CAD build for the part. Positions are in the model's coordinates, mm. A direction names the side the tool comes from. Round coordinates to 2 decimals unless told otherwise and drop trailing zeros. Loops run counter-clockwise (first coordinate to the right, second up) from the corner with the lowest first, then second, coordinate; pieces in that order, holes last.
```python
from build123d import *

# Parameters (mm, degrees)
F0_W     = 1.524
F0_H     = 6.35
F0_W_2   = 6.35
F0_H_2   = 1.524
F1_DEPTH = 1.524


with BuildPart() as f1:
    # F0 (on Front) → F1 (new body)
    with BuildSketch(Plane.XZ):
        Polygon((30.226, 19.05), (30.226, 25.4), (25.4, 25.4), (25.4, 21.0894770619), (25.4, -21.0894770619), (25.4, -25.4), (21.0894770619, -25.4), (-21.0894770619, -25.4), (-25.4, -25.4), (-25.4, -21.0894770619), (-25.4, 21.0894770619), (-25.4, 25.4), (-30.226, 25.4), (-30.226, 19.05), (-30.226, 12.7), (-30.226, -12.7), (-30.226, -19.05), (-30.226, -31.75), (-19.05, -31.75), (-12.7, -31.75), (12.7, -31.75), (19.05, -31.75), (30.226, -31.75), (30.226, -19.05), (30.226, -12.7), (30.226, 12.7), align=None)
        with Locations((-30.988, -15.875)):
            Rectangle(F0_W, F0_H)
        with Locations((-15.875, -32.512)):
            Rectangle(F0_W_2, F0_H_2)
        with Locations((15.875, -32.512)):
            Rectangle(F0_W_2, F0_H_2)
        Polygon((25.4, -25.4), (25.4, -21.0894770619), (4.3105229381, 0), (0, -4.3105229381), (21.0894770619, -25.4), align=None)
        Polygon((4.3105229381, 0), (0, 4.3105229381), (-4.3105229381, 0), (0, -4.3105229381), align=None)
        Polygon((25.4, 21.0894770619), (25.4, 25.4), (21.0894770619, 25.4), (0, 4.3105229381), (4.3105229381, 0), align=None)
        Polygon((-4.3105229381, 0), (0, 4.3105229381), (-21.0894770619, 25.4), (-25.4, 25.4), (-25.4, 21.0894770619), align=None)
        Polygon((0, -4.3105229381), (-4.3105229381, 0), (-25.4, -21.0894770619), (-25.4, -25.4), (-21.0894770619, -25.4), align=None)
        Polygon((-19.05, 31.75), (-21.0894770619, 31.75), (-25.4, 31.75), (-30.226, 31.75), (-30.226, 25.4), (-25.4, 25.4), (-21.0894770619, 25.4), (-19.05, 25.4), (-19.05, 26.924), (-12.7, 26.924), (-12.7, 25.4), (0, 25.4), (0, 31.75), (-12.7, 31.75), (-12.7, 30.226), (-19.05, 30.226), align=None)
        with Locations((-15.875, 26.162)):
            Rectangle(F0_W_2, F0_H_2)
        Polygon((30.226, 25.4), (30.226, 31.75), (25.4, 31.75), (21.0894770619, 31.75), (19.05, 31.75), (19.05, 30.226), (12.7, 30.226), (12.7, 31.75), (0, 31.75), (0, 25.4), (12.7, 25.4), (12.7, 26.924), (19.05, 26.924), (19.05, 25.4), (21.0894770619, 25.4), (25.4, 25.4), align=None)
        with Locations((15.875, 26.162)):
            Rectangle(F0_W_2, F0_H_2)
        with Locations((15.875, 30.988)):
            Rectangle(F0_W_2, F0_H_2)
        Polygon((25.4, 31.75), (30.226, 31.75), (30.226, 38.1), (30.226, 44.45), (30.226, 69.85), (30.226, 76.2), (30.226, 88.9), (19.05, 88.9), (12.7, 88.9), (-12.7, 88.9), (-19.05, 88.9), (-30.226, 88.9), (-30.226, 76.2), (-30.226, 69.85), (-30.226, 44.45), (-30.226, 38.1), (-30.226, 31.75), (-25.4, 31.75), (-25.4, 36.0605229381), (-25.4, 78.2394770619), (-25.4, 82.55), (-21.0894770619, 82.55), (21.0894770619, 82.55), (25.4, 82.55), (25.4, 78.2394770619), (25.4, 36.0605229381), align=None)
        Polygon((-21.0894770619, 31.75), (0, 52.8394770619), (-4.3105229381, 57.15), (-25.4, 36.0605229381), (-25.4, 31.75), align=None)
        Polygon((-4.3105229381, 57.15), (0, 52.8394770619), (4.3105229381, 57.15), (0, 61.4605229381), align=None)
        Polygon((0, 61.4605229381), (4.3105229381, 57.15), (25.4, 78.2394770619), (25.4, 82.55), (21.0894770619, 82.55), align=None)
        Polygon((21.0894770619, 31.75), (25.4, 31.75), (25.4, 36.0605229381), (4.3105229381, 57.15), (0, 52.8394770619), align=None)
        Polygon((-25.4, 78.2394770619), (-4.3105229381, 57.15), (0, 61.4605229381), (-21.0894770619, 82.55), (-25.4, 82.55), align=None)
        with Locations((15.875, 89.662)):
            Rectangle(F0_W_2, F0_H_2)
        with Locations((-15.875, 89.662)):
            Rectangle(F0_W_2, F0_H_2)
        with Locations((-30.988, 73.025)):
            Rectangle(F0_W, F0_H)
        with Locations((30.988, 73.025)):
            Rectangle(F0_W, F0_H)
        with Locations((30.988, -15.875)):
            Rectangle(F0_W, F0_H)
        with Locations((-15.875, 30.988)):
            Rectangle(F0_W_2, F0_H_2)
    extrude(amount=F1_DEPTH)


solid = f1.part
```
Item 1: Two-plate mould, pull along Z, no slides. Class faces 3 (the flat face through (0, -1.524, 29)), 4 (the flat face through (14.71, -0.75, 67.55)): released by +Z, released by -Z, zero draft, split by the parting line, or undercut.
Answers follow:
face 3: zero draft
face 4: undercut
Item 2: Probe line 1 (X direction, y = -0.6, z = 0); line 2 (X direction, y = -0.55, z = 55); line 3 (Z direction, x = 23.5, y = -1.15). List the from-to ranges inside material, lowest first.
Answers follow:
line 1: x = -30.23 to -25.4, -4.31 to 4.31, 25.4 to 30.23
line 2: x = -30.23 to -25.4, -6.46 to 6.46, 25.4 to 30.23
line 3: z = -31.75 to -19.19, 19.19 to 37.96, 76.34 to 88.9
Item 3: Cut at D-D, the plane z = 33. Give the cut face in (x, y), plus the area to 3 significant figures.
Answers follow:
outline: (-30.23, -1.52) - (-19.84, -1.52) - (-19.84, 0) - (-30.23, 0) - close; (19.84, -1.52) - (30.23, -1.52) - (30.23, 0) - (19.84, 0) - close
area: 31.7 mm2
Item 4: Flat gauge pins, fed straight in: P1, Ø0.8, axis at x = -23.5, y = -1, coming from the -Z side; P2, Ø0.8, axis at x = 31.5, y = -0.5, coming from the -Z side; P3, Ø0.8, axis at y = -0.5, z = -23, coming from the -X side. Where does each tip first touch, or does it go through?
Answers follow:
P1: stops at z = -31.75
P2: stops at z = -19.05
P3: stops at x = -30.23
Item 5: 3-axis set-ups, long thin cutter, end or side, ignore diameter. For faces 1 (the flat face through (10.4, -0.75, -14.71)), 2 (the flat face through (0, 0, 29)): which of +Z, -Z, +X, -X, +Y, -Y reach the whole face in a straight line?
Answers follow:
face 1: +Y, -Y
face 2: +Z, -Z, +X, -X, +Y
Item 6: Cut at B-B, the plane z = 12. Give the cut face in (x, y).
Answers follow:
outline: (-30.23, -1.52) - (-25.4, -1.52) - (-25.4, 0) - (-30.23, 0) - close; (-16.31, -1.52) - (-7.69, -1.52) - (-7.69, 0) - (-16.31, 0) - close; (7.69, -1.52) - (16.31, -1.52) - (16.31, 0) - (7.69, 0) - close; (25.4, -1.52) - (30.23, -1.52) - (30.23, 0) - (25.4, 0) - close
Item 7: Cut at A-A, the plane x = -8.5. Give the cut face in (y, z), plus the area to 3 significant figures.
Answers follow:
outline: (-1.52, -31.75) - (0, -31.75) - (0, -25.4) - (-1.52, -25.4) - close; (-1.52, -12.81) - (0, -12.81) - (0, -4.19) - (-1.52, -4.19) - close; (-1.52, 4.19) - (0, 4.19) - (0, 12.81) - (-1.52, 12.81) - close; (-1.52, 25.4) - (0, 25.4) - (0, 31.75) - (-1.52, 31.75) - close; (-1.52, 44.34) - (0, 44.34) - (0, 52.96) - (-1.52, 52.96) - close; (-1.52, 61.34) - (0, 61.34) - (0, 69.96) - (-1.52, 69.96) - close; (-1.52, 82.55) - (0, 82.55) - (0, 88.9) - (-1.52, 88.9) - close
area: 81.6 mm2
Item 8: Cut at C-C, the plane x = 2. Give the cut face in (y, z).
Answers follow:
outline: (-1.52, -31.75) - (0, -31.75) - (0, -25.4) - (-1.52, -25.4) - close; (-1.52, -6.31) - (0, -6.31) - (0, 6.31) - (-1.52, 6.31) - close; (-1.52, 25.4) - (0, 25.4) - (0, 31.75) - (-1.52, 31.75) - close; (-1.52, 50.84) - (0, 50.84) - (0, 63.46) - (-1.52, 63.46) - close; (-1.52, 82.55) - (0, 82.55) - (0, 88.9) - (-1.52, 88.9) - close
